Work out the finished part from the listing and answer in its coordinate system (mm). A direction names the side the tool comes from. Round coordinates to 2 decimals unless told otherwise and drop trailing zeros. Loops run counter-clockwise (first coordinate to the right, second up) from the corner with the lowest first, then second, coordinate; pieces in that order, holes last. Notation, with made-up numbers: (55.5, 86.25) - (114.5, 86.25) arc R29 ccw to (114.5, 107.25) - close; hole circle Ø3 at (41.25, 55). An arc over 180 degrees is marked (long way). Return JSON: item names as keys, results as strings.
from build123d import *

# Parameters (mm, degrees)
SKETCH1_W             = 44.196
SKETCH1_H             = 31.75
BOSS_EXTRUDE1_DEPTH   = 6.35
SKETCH3_W             = 2.54
SKETCH3_H             = 31.75
BOSS_EXTRUDE3_DEPTH   = 5.08
F_3_0MM_DOWEL_HOLE1_D = 3
CHAMFER1_SIZE         = 0.254
FILLET2_R             = 3.81
BOSS_EXTRUDE4_DEPTH   = 5.08
SKETCH7_W             = 16.51
SKETCH7_H             = 2.54
BOSS_EXTRUDE5_DEPTH   = 1.27
FILLET3_R             = 2.54


with BuildPart() as part:
    # Sketch1 → Boss-Extrude1 (new body)
    with BuildSketch(Plane(origin=(0, 0, 0), x_dir=(1, 0, 0), z_dir=(0, 1, 0))):
        with Locations((22.098, 15.875)):
            Rectangle(SKETCH1_W, SKETCH1_H)
    extrude(amount=BOSS_EXTRUDE1_DEPTH)

    # Sketch3 → Boss-Extrude3 (add)
    with BuildSketch(Plane.XZ):
        with Locations((19.05, -15.875)):
            Rectangle(SKETCH3_W, SKETCH3_H)
    extrude(amount=BOSS_EXTRUDE3_DEPTH)

    # Ø3.0mm Dowel Hole1 (through all)
    with Locations(Plane(origin=(0, 6.35, 0), x_dir=(1, 0, 0), z_dir=(0, 1, 0))):
        with Locations((5.08, 15.875), (12.7, 15.875)):
            Hole(F_3_0MM_DOWEL_HOLE1_D / 2)

    # Chamfer1
    chamfer1_edges = [part.edges().sort_by_distance(p)[0] for p in [
        (14.2, 0, -15.875),
        (14.2, 6.35, -15.875),
        (6.58, 0, -15.875),
        (6.58, 6.35, -15.875),
    ]]
    chamfer(chamfer1_edges, length=CHAMFER1_SIZE)

    # Fillet2
    fillet2_edges = [part.edges().sort_by_distance(p)[0] for p in [
        (0, 3.175, 0),
        (0, 3.175, -31.75),
    ]]
    fillet(fillet2_edges, radius=FILLET2_R)

    # Sketch6 → Boss-Extrude4 (add)
    with BuildSketch(Plane(origin=(44.196, 0, 0), x_dir=(0, 0, -1), z_dir=(1, 0, 0))):
        Polygon((0, 6.35), (0, -21.59), (31.75, -21.59), (31.75, 6.35), (24.13, 6.35), (24.13, -13.97), (7.62, -13.97), (7.62, 6.35), align=None)
    extrude(amount=BOSS_EXTRUDE4_DEPTH)

    # Sketch7 → Boss-Extrude5 (add)
    with BuildSketch(Plane.ZY.offset(-44.196)):
        with Locations((-15.875, -20.32)):
            Rectangle(SKETCH7_W, SKETCH7_H)
    extrude(amount=BOSS_EXTRUDE5_DEPTH)

    # Fillet3
    fillet3_edges = [part.edges().sort_by_distance(p)[0] for p in [
        (42.926, -21.59, -15.875),
    ]]
    fillet(fillet3_edges, radius=FILLET3_R - 0.0001)  # a hair under: the kernel refuses the full size


solid = part.part
1) A tool of negligible diameter and unlimited length cuts with its end or side. For faces 4 (the flat face through (47, -4, -24.13)), 5 (the flat face through (44, -20, -7.62)), 6 (the flat face through (19, -5.08, -16)), from which of +Z, -Z, +X, -X, +Y, -Y can it reach the whole face along a straight path? Write none if from no direction.
Verdict:
{"face 4": "+X, +Y", "face 5": "+Z, -X, -Y", "face 6": "+Z, -Z, -X, -Y"}
2) Section D-D (y = -13) is taken. Give the vertices of the cut face in (x, z).
Verdict:
{"outline": "(44.2, -31.75) - (49.28, -31.75) - (49.28, -24.13) - (44.2, -24.13) - close; (44.2, -7.62) - (49.28, -7.62) - (49.28, 0) - (44.2, 0) - close"}
3) Flat-ended cylindrical pins translate along their axes: pin 1 (8 mm diameter, centred on y = -13.5, z = -25, fed in from -X); pin 2 (4 mm diameter, centred on x = 47.5, z = -12.5, fed in from +Y); pin 3 (7 mm diameter, centred on x = 30, z = -21, fed in from -Y). Find the tip coordinate at first contact, or state that the pin passes through.
Verdict:
{"pin 1": "stops at x = 44.2", "pin 2": "stops at y = -13.97", "pin 3": "stops at y = 0"}
4) Section A-A (y = -2.5) is taken. Give the vertices of the cut face in (x, z).
Verdict:
{"outline": "(17.78, -31.75) - (20.32, -31.75) - (20.32, 0) - (17.78, 0) - close; (44.2, -31.75) - (49.28, -31.75) - (49.28, -24.13) - (44.2, -24.13) - close; (44.2, -7.62) - (49.28, -7.62) - (49.28, 0) - (44.2, 0) - close"}
5) Determine the mould class of faces 1 (the flat face through (44.196, 3, -16)), 2 (the flat face through (47, -4, -7.62)), 3 (the cylindrical face through (6.186, 3.134, -16.889)) for opening direction X: pulls with the +X half, pulls with the -X half, needs draft (parallel to the pull), parting line crosses it, or undercut.
Verdict:
{"face 1": "pulls with the +X half", "face 2": "needs draft", "face 3": "undercut"}
6) Section B-B (x = 12.7) is taken. Give the vertices of the cut face in (y, z) (3 decimals), and give its area (3 significant figures).
Verdict:
{"outline": "(0, -31.75) - (6.35, -31.75) - (6.35, -17.629) - (6.096, -17.375) - (0.254, -17.375) - (0, -17.629) - close; (0, -14.121) - (0.254, -14.375) - (6.096, -14.375) - (6.35, -14.121) - (6.35, 0) - (0, 0) - close", "area": "182 mm2"}
7) Find the intervals of material crossed by L1, parallel to Z at x = 46.5, y = -11; L2, parallel to Z at x = 5.08, y = 1.95 (3 decimals); L3, parallel to Y at x = 38, z = -17, in increasing order.
Verdict:
{"L1": "z = -31.75 to -24.13, -7.62 to 0", "L2": "z = -31.75 to -17.375, -14.375 to 0", "L3": "y = 0 to 6.35"}
